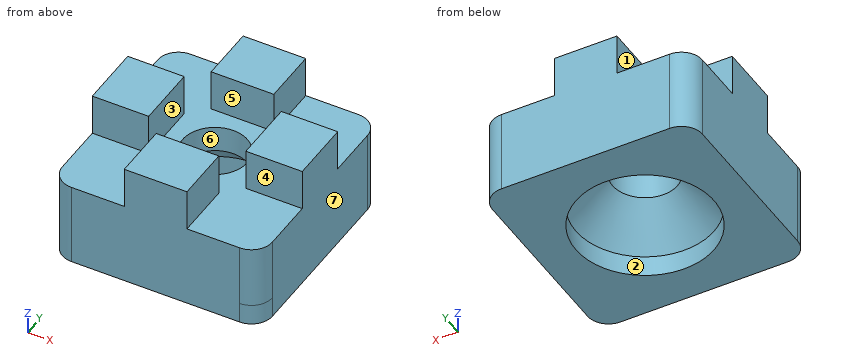
```python
from build123d import *

# Parameters (mm, degrees)
F0_R     = 3.1
F0_W     = 5.4
F0_H     = 6
F0_W_2   = 6
F0_H_2   = 5.4
F1_DEPTH = 6
F2_DEPTH = 10
F3_R     = 2
F4_SIZE  = 3.5
F5_DEPTH = 2


# Not quite as in the source:
# - a feature names something its author has since deleted; it is built from what else it names


with BuildPart() as f1:
    # F0 (on Top) → F1 (new body)
    with BuildSketch(Plane.XY):
        Polygon((-7.9959459106, 7.05), (-7.9959459106, 0), (-0.9459459106, 0), (-0.9459459106, 5.4), (5.0540540894, 5.4), (5.0540540894, 0), (12.1040540894, 0), (12.1040540894, 7.05), (6.7040540894, 7.05), (6.7040540894, 13.05), (12.1040540894, 13.05), (12.1040540894, 20.1), (5.0540540894, 20.1), (5.0540540894, 14.7), (-0.9459459106, 14.7), (-0.9459459106, 20.1), (-7.9959459106, 20.1), (-7.9959459106, 13.05), (-2.5959459106, 13.05), (-2.5959459106, 7.05), align=None)
        with Locations((2.0540540894, 10.05)):
            Circle(F0_R, mode=Mode.SUBTRACT)
        with Locations((9.4040540894, 10.05)):
            Rectangle(F0_W, F0_H)
        with Locations((-5.2959459106, 10.05)):
            Rectangle(F0_W, F0_H)
        with Locations((2.0540540894, 17.4)):
            Rectangle(F0_W_2, F0_H_2)
        with Locations((2.0540540894, 2.7)):
            Rectangle(F0_W_2, F0_H_2)
    extrude(amount=F1_DEPTH)

    # F0 (on Top) → F2 (join)
    with BuildSketch(Plane.XY):
        with Locations((2.0540540894, 17.4)):
            Rectangle(F0_W_2, F0_H_2)
        with Locations((-5.2959459106, 10.05)):
            Rectangle(F0_W, F0_H)
        with Locations((2.0540540894, 2.7)):
            Rectangle(F0_W_2, F0_H_2)
        with Locations((9.4040540894, 10.05)):
            Rectangle(F0_W, F0_H)
    extrude(amount=F2_DEPTH)

    # F3
    f3_edges = [f1.edges().sort_by_distance(p)[0] for p in [
        (-7.995946, 0, 3),
        (12.104054, 0, 3),
        (12.104054, 20.1, 3),
        (-7.995946, 20.1, 3),
    ]]
    fillet(f3_edges, radius=F3_R)

    # F4
    f4_edges = [f1.edges().sort_by_distance(p)[0] for p in [
        (-1.045946, 10.05, 0),
    ]]
    chamfer(f4_edges, length=F4_SIZE)

    # F5 (add): a face of the model
    f5_faces = [f1.faces().sort_by_distance(p)[0] for p in [
        (-4.8302028367, 10.05, 0),
    ]]
    extrude(f5_faces, amount=F5_DEPTH)


solid = f1.part
```
Here's how the part is built. I have some questions about the finished solid (model axes, mm). Face numbers are marked on the shaded views. A direction names the side the tool comes from. Give positions to 0.01 mm unless a question says otherwise; leave off trailing zeros. Write each loop counter-clockwise with the first axis right and the second up, starting at its lowest first coordinate (ties: lowest second). Pieces come first, ordered by that corner, then holes. Notation, with made-up numbers: (77, 62) -> (100, 62) arc R32 ccw to (100, 89) -> close; hole circle Ø8 at (68.5, 44). An arc over 180 degrees is marked (long way). Write each question's results on one line, items separated by ' | '.
Item 1: On a 3-axis mill with a long thin cutter (end or side, diameter ignored), from which of +Z, -Z, +X, -X, +Y, -Y can I reach the whole of each face in a straight line? I mean the marked faces 1, 2, 3 and 4. Say none if no direction works.
Output:
face 1: +Z, -X, +Y, -Y | face 2: -Z | face 3: +Z, +Y, -Y | face 4: +Z, +X, -X, -Y
Item 2: Suppose I cut it at A-A on y = 10.05. Write out the boundary of the cut face in (x, z), plus the area to 3 significant figures.
Output:
outline: (-8, -2) -> (-4.55, -2) -> (-4.55, 0) -> (-1.05, 3.5) -> (-1.05, 6) -> (-2.6, 6) -> (-2.6, 10) -> (-8, 10) -> close; (5.15, 3.5) -> (8.65, 0) -> (8.65, -2) -> (12.1, -2) -> (12.1, 10) -> (6.7, 10) -> (6.7, 6) -> (5.15, 6) -> close | area: 128 mm^2
Item 3: Suppose I cut it at B-B on z = 4.25. Write out the boundary of the cut face in (x, y).
Output:
outline: (-8, 2) arc R2 ccw to (-6, 0) -> (10.1, 0) arc R2 ccw to (12.1, 2) -> (12.1, 18.1) arc R2 ccw to (10.1, 20.1) -> (-6, 20.1) arc R2 ccw to (-8, 18.1) -> close; hole circle Ø6.2 at (2.05, 10.05)
Item 4: We'd pull the mould along X, two halves only. Please class the marked faces 5, 6 and 7: pulls with the +X half, pulls with the -X half, needs draft (parallel to the pull), parting line crosses it, or undercut.
Output:
face 5: needs draft | face 6: undercut | face 7: pulls with the +X half
Item 5: If I drill on L1, parallel to Y at x = -1, z = 0.25; L2, parallel to X at y = 17.75, z = 8; L3, parallel to Z at x = 9, y = 16.75, over which ranges is the centre line in solid material (lowest first)?
Output:
L1: y = 0 to 4.48, 15.62 to 20.1 | L2: x = -0.95 to 5.05 | L3: z = -2 to 6
Item 6: For pin 1 Ø3 at (x, y) = (0, 14.5) entering from -Z; pin 2 Ø3 at (y, z) = (18.5, 8) entering from -X; pin 3 Ø1.2 at (x, z) = (10, 8) entering from +Y, each with a flat end and sliding along its axis, tell me the tip position at first contact or that it passes through.
Output:
pin 1: stops at z = 0.2 | pin 2: stops at x = -0.95 | pin 3: stops at y = 13.05
Item 7: Suppose I cut it at C-C on y = 3. Write out the boundary of the cut face in (x, z).
Output:
outline: (-8, -2) -> (12.1, -2) -> (12.1, 6) -> (5.05, 6) -> (5.05, 10) -> (-0.95, 10) -> (-0.95, 6) -> (-8, 6) -> close
Item 8: Suppose I cut it at D-D on z = 1.25. Write out the boundary of the cut face in (x, y).
Output:
outline: (-8, 2) arc R2 ccw to (-6, 0) -> (10.1, 0) arc R2 ccw to (12.1, 2) -> (12.1, 18.1) arc R2 ccw to (10.1, 20.1) -> (-6, 20.1) arc R2 ccw to (-8, 18.1) -> close; hole circle Ø10.7 at (2.05, 10.05)
